Source: CAD feature listing. Evaluate the final solid. Frame: model axes, mm. A direction names the side the tool comes from. Coordinates: 2 decimals unless noted, no trailing zeros. Order: outer loops, then holes, each group sorted by start corner. A loop starts at its lowest first (then second) coordinate and runs counter-clockwise, first axis right, second up. Notation, with made-up numbers: (58, 48.5) -> (66, 48.5) arc R22 ccw to (66, 57.5) -> close; hole circle Ø8 at (56, -4.75). An arc over 180 degrees is marked (long way). Put each result on its own line as item: value.
from build123d import *

# Parameters (mm, degrees)
BASE_FLANGE1_DEPTH      = 50.8
CUT_EXTRUDE1_DEPTH      = 69.790674268
CUT_EXTRUDE1_DEPTH_BACK = 69.790674268
SKETCH3_R               = 2.4892


# Sheet-metal steps are written as plain solids
with BuildPart() as part:
    # Sketch1 → Base-Flange1 (new body)
    with BuildSketch(Plane.XY):
        with BuildLine():
            Line((-42.95775, -7.9375), (-42.95775, 7.1755))
            ThreePointArc((-42.95775, 7.1755), (-42.734565367, 7.714315367), (-42.19575, 7.9375))
            Line((-42.19575, 7.9375), (42.19575, 7.9375))
            ThreePointArc((42.19575, 7.9375), (42.734565367, 7.714315367), (42.95775, 7.1755))
            Line((42.95775, 7.1755), (42.95775, -7.9375))
            Line((42.95775, -7.9375), (45.24375, -7.9375))
            Line((45.24375, -7.9375), (45.24375, 7.1755))
            ThreePointArc((45.24375, 7.1755), (44.351011469, 9.330761469), (42.19575, 10.2235))
            Line((42.19575, 10.2235), (-42.19575, 10.2235))
            ThreePointArc((-42.19575, 10.2235), (-44.351011469, 9.330761469), (-45.24375, 7.1755))
            Line((-45.24375, 7.1755), (-45.24375, -7.9375))
            Line((-45.24375, -7.9375), (-42.95775, -7.9375))
        make_face()
    extrude(amount=BASE_FLANGE1_DEPTH)

    # Sketch3 → Cut-Extrude1 (cut, two sides: drawn at the far end of the back side and taken through both)
    with BuildSketch(Plane(origin=(0, 0, 0), x_dir=(0, 0, -1), z_dir=(1, 0, 0)).offset(-CUT_EXTRUDE1_DEPTH_BACK)):
        with Locations((-6.35, 0.6985)):
            Circle(SKETCH3_R)
        with Locations((-19.05, 0.6985)):
            Circle(SKETCH3_R)
        with Locations((-31.75, 0.6985)):
            Circle(SKETCH3_R)
        with Locations((-44.45, 0.6985)):
            Circle(SKETCH3_R)
    extrude(amount=CUT_EXTRUDE1_DEPTH + CUT_EXTRUDE1_DEPTH_BACK, mode=Mode.SUBTRACT)


solid = part.part
1. Set-up query: faces 4 (the flat face through (-42.958, 0, 25)), 5 (the flat face through (1, 10.224, 25)). Return all of +Z, -Z, +X, -X, +Y, -Y with unobstructed straight access to the full face (end or side cutting, diameter ignored); none if empty.
Numbers:
face 4: +Z, -Z, -Y
face 5: +Z, -Z, +X, -X, +Y
2. Ray query, line 1 along X through (y, z) = (-3, 20); line 2 along Y through (x, z) = (16, 44); line 3 along Y through (x, z) = (-44.5, 31.75). Return the intervals inside material, ascending.
Numbers:
line 1: x = -45.24 to -42.96, 42.96 to 45.24
line 2: y = 7.94 to 10.22
line 3: y = -7.94 to -1.79, 3.19 to 9.17
3. Cut plane A-A on z = 44.45. Output: boundary loops of the cut face in (x, y), plus the area to 3 significant figures.
Numbers:
outline: (-45.24, -7.94) -> (-42.96, -7.94) -> (-42.96, -1.79) -> (-45.24, -1.79) -> close; (-45.24, 3.19) -> (-42.96, 3.19) -> (-42.96, 7.18) arc R0.76 cw to (-42.2, 7.94) -> (42.2, 7.94) arc R0.76 cw to (42.96, 7.18) -> (42.96, 3.19) -> (45.24, 3.19) -> (45.24, 7.18) arc R3.05 ccw to (42.2, 10.22) -> (-42.2, 10.22) arc R3.05 ccw to (-45.24, 7.18) -> close; (42.96, -7.94) -> (45.24, -7.94) -> (45.24, -1.79) -> (42.96, -1.79) -> close
area: 253 mm2
4. Cut plane D-D on x = -25. Output: boundary loops of the cut face in (y, z).
Numbers:
outline: (7.94, 0) -> (10.22, 0) -> (10.22, 50.8) -> (7.94, 50.8) -> close
5. Cut plane B-B on z = 12.5. Output: boundary loops of the cut face in (x, y), plus the area to 3 significant figures.
Numbers:
outline: (-45.24, -7.94) -> (-42.96, -7.94) -> (-42.96, 7.18) arc R0.76 cw to (-42.2, 7.94) -> (42.2, 7.94) arc R0.76 cw to (42.96, 7.18) -> (42.96, -7.94) -> (45.24, -7.94) -> (45.24, 7.18) arc R3.05 ccw to (42.2, 10.22) -> (-42.2, 10.22) arc R3.05 ccw to (-45.24, 7.18) -> close
area: 276 mm2
6. Cut plane C-C on z = 7. Output: boundary loops of the cut face in (x, y).
Numbers:
outline: (-45.24, -7.94) -> (-42.96, -7.94) -> (-42.96, -1.7) -> (-45.24, -1.7) -> close; (-45.24, 3.1) -> (-42.96, 3.1) -> (-42.96, 7.18) arc R0.76 cw to (-42.2, 7.94) -> (42.2, 7.94) arc R0.76 cw to (42.96, 7.18) -> (42.96, 3.1) -> (45.24, 3.1) -> (45.24, 7.18) arc R3.05 ccw to (42.2, 10.22) -> (-42.2, 10.22) arc R3.05 ccw to (-45.24, 7.18) -> close; (42.96, -7.94) -> (45.24, -7.94) -> (45.24, -1.7) -> (42.96, -1.7) -> close
7. First-contact query: pin 1 (8 mm diameter, centred on y = 0.7, z = 6.35, fed in from -X); pin 2 (1 mm diameter, centred on x = 30.5, z = 8, fed in from -Y); pin 3 (4 mm diameter, centred on y = 0.7, z = 31.75, fed in from -X). Flat tips, straight axial feed; report the tip coordinate or a pass-through.
Numbers:
pin 1: stops at x = -45.24
pin 2: stops at y = 7.94
pin 3: passes through
8. Pull-direction query (Y, two-part tool) for faces 1 (the cylindrical face through (-44.12, -0.25, 42.15)), 2 (the cylindrical face through (44.37, 9.31, 25.04)), 3 (the flat face through (42.958, 0, 25)); classes: pulls with the +Y half, pulls with the -Y half, needs draft (parallel to the pull), parting line crosses it, or undercut.
Numbers:
face 1: undercut
face 2: pulls with the +Y half
face 3: needs draft
